```python
from build123d import *

# Parameters (mm, degrees)
CIRCLE006_R        = 20
EXTRUSION023_DEPTH = 1.371598
RECTANGLE013_W     = 20
RECTANGLE013_H     = 20
EXTRUSION022_DEPTH = 1.371598


with BuildPart() as extrusion023:
    # Circle006 (on Rectangle) → Extrusion023 (new body)
    with BuildSketch(Plane(origin=(-782.323582, -43.476219, 16.366052), x_dir=(0, -1, 0), z_dir=(-1, 0, 0))):
        Circle(CIRCLE006_R)
    extrude(amount=-EXTRUSION023_DEPTH)


with BuildPart() as cut004006005004002008019023005025006:
    # Rectangle013 → Extrusion022 (new body)
    with BuildSketch(Plane(origin=(-782.323582, -23.476219, -3.633948), x_dir=(0, -1, 0), z_dir=(-1, 0, 0))):
        with Locations((10, 10)):
            Rectangle(RECTANGLE013_W, RECTANGLE013_H)
    extrude(amount=-EXTRUSION022_DEPTH)

    # Cut004006005004002008019023005025006: cut Extrusion023
    add(extrusion023.part, mode=Mode.SUBTRACT)


solid = cut004006005004002008019023005025006.part
```
For this review, take the finished solid that the model builds, in its own axes (mm). Round coordinates to 2 decimals unless told otherwise and drop trailing zeros. Write each loop counter-clockwise with the first axis right and the second up, starting at its lowest first coordinate (ties: lowest second). Pieces come first, ordered by that corner, then holes.
1) Take a section at B-B on y = -39.25. Give the boundary of the cut face in (x, z).
Answer below:
outline: (-782.32, -3.63) - (-780.95, -3.63) - (-780.95, -3.18) - (-782.32, -3.18) - close
2) Take a section at A-A on x = -781.2. Give the boundary of the cut face in (y, z), then the cut area to 3 significant figures.
Answer below:
outline: (-43.48, -3.63) - (-23.48, -3.63) - (-23.48, 16.37) arc R20 cw to start
area: 85.8 mm2
3) Take a section at C-C on z = 6. Give the boundary of the cut face in (x, y), then the cut area to 3 significant figures.
Answer below:
outline: (-782.32, -26.37) - (-780.95, -26.37) - (-780.95, -23.48) - (-782.32, -23.48) - close
area: 3.97 mm2
4) For line 1 along Y through (x, z) = (-781.65, 5.25); line 2 along Y through (x, z) = (-781.9, 1.5); line 3 along Z through (x, y) = (-781.65, -36.5), list the stretches that pass through material, from the lowest coordinate up.
Answer below:
line 1: y = -26.85 to -23.48
line 2: y = -30.1 to -23.48
line 3: z = -3.63 to -2.38
